Work out the finished part from the listing and answer in its coordinate system (mm). A direction names the side the tool comes from. Round coordinates to 2 decimals unless told otherwise and drop trailing zeros. Write each loop counter-clockwise with the first axis right and the second up, starting at its lowest first coordinate (ties: lowest second). Pieces come first, ordered by that corner, then holes. Notation, with made-up numbers: (-9, -22) -> (24, -22) arc R13 cw to (24, -5) -> close; hole circle Ø3 at (5, -21). An arc over 180 degrees is marked (long way). One line per question, with ' | ' between items. Start each with the question number.
```python
from build123d import *

# Parameters (mm, degrees)
SKETCH1_W           = 75.565
SKETCH1_H           = 37.465
SKETCH1_W_2         = 72.39
SKETCH1_H_2         = 34.29
BOSS_EXTRUDE1_DEPTH = 19.05
SKETCH2_W           = 75.565
SKETCH2_H           = 37.465
BOSS_EXTRUDE2_DEPTH = 1.5875
SKETCH3_W           = 6.35
SKETCH3_H           = 6.35
CUT_EXTRUDE1_DEPTH  = 19.05


with BuildPart() as part:
    # Sketch1 → Boss-Extrude1 (new body)
    with BuildSketch(Plane(origin=(0, 0, 0), x_dir=(1, 0, 0), z_dir=(0, 1, 0))):
        with Locations((36.195, 17.145)):
            Rectangle(SKETCH1_W, SKETCH1_H)
        with Locations((36.195, 17.145)):
            Rectangle(SKETCH1_W_2, SKETCH1_H_2, mode=Mode.SUBTRACT)
    extrude(amount=BOSS_EXTRUDE1_DEPTH)

    # Sketch2 → Boss-Extrude2 (add)
    with BuildSketch(Plane.XZ):
        with Locations((36.195, -17.145)):
            Rectangle(SKETCH2_W, SKETCH2_H)
    extrude(amount=BOSS_EXTRUDE2_DEPTH)

    # Sketch3 → Cut-Extrude1 (cut)
    with BuildSketch(Plane(origin=(0, 19.05, 0), x_dir=(1, 0, 0), z_dir=(0, 1, 0))):
        with Locations((1.5875, 32.7025)):
            Rectangle(SKETCH3_W, SKETCH3_H)
    extrude(amount=-CUT_EXTRUDE1_DEPTH, mode=Mode.SUBTRACT)


solid = part.part
```
(1) A cutting plane is placed at C-C, the plane z = -9.5. Determine the outline of the cut face in (x, y).
(2) A cutting plane is placed at B-B, the plane x = 18. Determine the outline of the cut face in (y, z).
(3) Consider L1, parallel to Z at x = 49.5, y = 5.75; L2, parallel to X at y = 18.25, z = -16; L3, parallel to Y at x = 47.5, z = -3.5. Determine where each line is inside the solid, lowest interval first.
(4) Given pin 1 Ø1.3 at (y, z) = (5, -35) entering from -X; pin 2 Ø1.7 at (x, y) = (-1, 5.5) entering from -Z; pin 3 Ø1 at (x, z) = (44, -8.5) entering from +Y, each flat-ended and moving along its own axis, determine where each tip first touches the part or whether it passes through.
(5) The mould has two halves that part along Z. Classify faces 6 (the flat face through (-1, 10, -29.528)), 7 (the flat face through (-1.587, 9, -13)), 8 (the flat face through (72.39, 9, -17)): +Z half, -Z half, draft (parallel to the pull), parting line (faces both ways), or undercut.
(6) For faces 1 (the flat face through (36, -1.588, -17)), 2 (the flat face through (38, 9, -34.29)), 3 (the flat face through (0, 9, -15)), 4 (the flat face through (36, 9, 0)), 5 (the flat face through (4.762, 10, -35)), determine the directions among +Z, -Z, +X, -X, +Y, -Y from which every point of the face is accessible in a straight line to the end or side of a thin tool.
(7) A cutting plane is placed at A-A, the plane y = 7. Determine the outline of the cut face in (x, z).
Returned:
1) outline: (-1.59, -1.59) -> (73.98, -1.59) -> (73.98, 19.05) -> (72.39, 19.05) -> (72.39, 0) -> (0, 0) -> (0, 19.05) -> (-1.59, 19.05) -> close
2) outline: (-1.59, -35.88) -> (19.05, -35.88) -> (19.05, -34.29) -> (0, -34.29) -> (0, 0) -> (19.05, 0) -> (19.05, 1.59) -> (-1.59, 1.59) -> close
3) L1: -35.88 to -34.29, 0 to 1.59 | L2: -1.59 to 0, 72.39 to 73.98 | L3: -1.59 to 0
4) pin 1: x = 4.76 | pin 2: z = -29.53 | pin 3: y = 0
5) face 6: -Z half | face 7: draft | face 8: undercut
6) face 1: +Z, -Z, +X, -X, -Y | face 2: -X, +Y | face 3: -Z, +Y | face 4: +Y | face 5: -Z, -X, +Y
7) outline: (-1.59, -29.53) -> (0, -29.53) -> (0, 0) -> (72.39, 0) -> (72.39, -34.29) -> (4.76, -34.29) -> (4.76, -35.88) -> (73.98, -35.88) -> (73.98, 1.59) -> (-1.59, 1.59) -> close
